```python
from build123d import *

# Parameters (mm, degrees)
F0_R     = 12.7
F1_DEPTH = 12.7


with BuildPart() as f1:
    # F0 (on Front) → F1 (new body)
    with BuildSketch(Plane.XZ):
        with BuildLine():
            ThreePointArc((18.932042, -16.933333), (23.727978, -9.063281), (25.4, 0))
            ThreePointArc((25.4, 0), (23.186922, 10.369507), (16.933333, 18.932042))
            ThreePointArc((16.933333, 18.932042), (9.063281, 23.727978), (0, 25.4))
            ThreePointArc((0, 25.4), (-10.369507, 23.186922), (-18.932042, 16.933333))
            ThreePointArc((-18.932042, 16.933333), (-23.727978, 9.063281), (-25.4, 0))
            ThreePointArc((-25.4, 0), (-23.186922, -10.369507), (-16.933333, -18.932042))
            ThreePointArc((-16.933333, -18.932042), (-9.063281, -23.727978), (0, -25.4))
            ThreePointArc((0, -25.4), (10.369507, -23.186922), (18.932042, -16.933333))
        make_face()
        Circle(F0_R, mode=Mode.SUBTRACT)
        with BuildLine():
            ThreePointArc((-18.932042, 16.933333), (-10.369507, 23.186922), (0, 25.4))
            Line((0, 25.4), (0, 38.1))
            Line((0, 38.1), (-18.932042, 16.933333))
        make_face()
        with BuildLine():
            ThreePointArc((16.933333, 18.932042), (23.186922, 10.369507), (25.4, 0))
            Line((25.4, 0), (38.1, 0))
            Line((38.1, 0), (16.933333, 18.932042))
        make_face()
        with BuildLine():
            Line((0, -38.1), (18.932042, -16.933333))
            ThreePointArc((18.932042, -16.933333), (10.369507, -23.186922), (0, -25.4))
            Line((0, -25.4), (0, -38.1))
        make_face()
        with BuildLine():
            Line((-38.1, 0), (-16.933333, -18.932042))
            ThreePointArc((-16.933333, -18.932042), (-23.186922, -10.369507), (-25.4, 0))
            Line((-25.4, 0), (-38.1, 0))
        make_face()
    extrude(amount=F1_DEPTH)


solid = f1.part
```
Part model, mm, in its own coordinate system. A direction names the side the tool comes from. Round coordinates to 2 decimals unless told otherwise and drop trailing zeros. Loops run counter-clockwise (first coordinate to the right, second up) from the corner with the lowest first, then second, coordinate; pieces in that order, holes last.
Item 1: Cut at D-D, the plane z = -23.5. Give the cut face in (x, y), then the cut area to 3 significant figures.
Item 2: 3-axis set-ups, long thin cutter, end or side, ignore diameter. For faces 1 (the face through (-32, -6, 0)), 2 (the face through (0, -6, 32)), 3 (the face through (32, -6, 0)): which of +Z, -Z, +X, -X, +Y, -Y reach the whole face in a straight line?
Item 3: Cut at B-B, the plane y = -3.25. Give the cut face in (x, z).
Item 4: Drill centre lines: line 1 (Z direction, x = 8.5, y = -2.5); line 2 (X direction, y = -11.75, z = -0.5); line 3 (Z direction, x = 3.5, y = -2.25). Where is each one in solid material? Low to high.
Item 5: Cut at A-A, the plane x = -10. Give the cut face in (y, z).
Item 6: Drop flat-ended pins along their axis: P1, Ø1.5, axis at x = 30, y = -10, coming from the -Z side; P2, Ø12, axis at x = -13.5, z = -27.5, coming from the -Y side; P3, Ø6, axis at y = -5, z = 20, coming from the +X side; P4, Ø4, axis at y = -5.5, z = 31.5, coming from the +X side. Give the stop position or say it passes through.
Item 7: Cut at C-C, the plane x = -2. Give the cut face in (y, z).
A:
1. outline: (-9.64, -12.7) - (13.06, -12.7) - (13.06, 0) - (-9.64, 0) - close
1. area: 288 mm2
2. face 1: +Z, -X, +Y, -Y
2. face 2: +Z, +X, +Y, -Y
2. face 3: -Z, +X, +Y, -Y
3. outline: (-38.1, 0) - (-16.93, -18.93) arc R25.4 ccw to (0, -25.4) - (0, -38.1) - (18.93, -16.93) arc R25.4 ccw to (25.4, 0) - (38.1, 0) - (16.93, 18.93) arc R25.4 ccw to (0, 25.4) - (0, 38.1) - (-18.93, 16.93) arc R25.4 ccw to (-25.4, 0) - close; hole circle Ø25.4 at (0, 0)
4. line 1: z = -28.6 to -9.44, 9.44 to 23.94
4. line 2: x = -37.54 to -12.69, 12.69 to 25.4
4. line 3: z = -34.19 to -12.21, 12.21 to 25.16
5. outline: (-12.7, -23.35) - (0, -23.35) - (0, -7.83) - (-12.7, -7.83) - close; (-12.7, 7.83) - (0, 7.83) - (0, 26.92) - (-12.7, 26.92) - close
6. P1: stops at z = 0
6. P2: stops at y = -12.7
6. P3: stops at x = 19.09
6. P4: stops at x = 0
7. outline: (-12.7, -25.32) - (0, -25.32) - (0, -12.54) - (-12.7, -12.54) - close; (-12.7, 12.54) - (0, 12.54) - (0, 35.86) - (-12.7, 35.86) - close
